Geometry: final body of the model. Coordinates: model frame, mm. A direction names the side the tool comes from. Round coordinates to 2 decimals unless told otherwise and drop trailing zeros. Loops run counter-clockwise (first coordinate to the right, second up) from the corner with the lowest first, then second, coordinate; pieces in that order, holes last. Notation, with made-up numbers: (41, 74) - (99, 74) arc R7 cw to (99, 82) - close; hole circle Ø8 at (-33.75, 52.25). An arc over 180 degrees is marked (long way). Return JSON: item names as keys, results as strings. Group by question number.
1. First-contact query: pin 1 Ø3.5 at (x, y) = (-2, 2.5) entering from -Z; pin 2 Ø0.5 at (y, z) = (6.5, -0.5) entering from -X. Flat tips, straight axial feed; report the tip coordinate or a pass-through.
2. Section B-B on x = -15. Return loops of the section in (y, z).
3. Set-up query: faces 1 (the face through (14.325, -1.312, 0.592)), 2 (the face through (0, 0, 0)), 3 (the face through (0, 0, 1.2)). Return all of +Z, -Z, +X, -X, +Y, -Y with unobstructed straight access to the full face (end or side cutting, diameter ignored); none if empty.
4. Draft query along X for faces 4 (the face through (-3, 5.817, 1)), 5 (the face through (-17.398, 5.697, 0.592)), 6 (the face through (-1, 6.717, 1)). Return one class per face: +X half, -X half, draft (parallel to the pull), parting line (faces both ways), or undercut.
5. Section A-A on x = 5. Return loops of the section in (y, z).
6. Section C-C on z = -1. Return loops of the section in (x, y), and give its area (3 significant figures).
7. Section D-D on y = -1.25. Return loops of the section in (x, z).
8. Material intervals for probe 1 along Y at (x, z) = (-9, 0.25); probe 2 along Y at (x, z) = (2, 2.5); probe 3 along Z at (x, y) = (9.5, -4.5), sorted ascending.
from build123d import *

# Parameters (mm, degrees)
EXTRUDE_1_DEPTH     = 1.2
CUT_EXTRUDE_START   = -1.2
CUT_EXTRUDE_1_DEPTH = 1.2
SKETCH_4_R          = 0.3
EXTRUDE_2_DEPTH     = 0.3
SKETCH_5_W          = 35.331764914
SKETCH_5_H          = 6.20328697
EXTRUDE_3_DEPTH     = 0.6


# Read off the part's stored shape, not the designer's step: Вырез-Вытянуть-Тонкостенный1
with BuildPart() as part:
    # Эскиз2 → Бобышка-Вытянуть1 (new body)
    with BuildSketch(Plane.XY):
        with BuildLine():
            Line((-18.718376773, 5.964639596), (-19.098029559, 5.834924894))
            Line((-19.098029559, 5.834924894), (-13.908113328, -6.217213911))
            Line((-13.908113328, -6.217213911), (10.163695982, -6.217213911))
            Line((10.163695982, -6.217213911), (19.098029559, 3.075246962))
            Line((19.098029559, 3.075246962), (18.818052215, 3.361181271))
            add(Edge.make_bspline(
                [(18.818052215, 3.361181271), (18.196335672, 3.797817809), (16.975433986, 4.6552669), (14.927683514, 5.553251977), (12.774537573, 6.124349252), (11.289757629, 6.1860932), (10.541386196, 6.217213911)],
                knots=[0, 0, 0, 0, 0.255164744, 0.501082157, 0.74853118, 1, 1, 1, 1], degree=3))
            Line((10.541386196, 6.217213911), (-16.231491208, 6.217213911))
            Line((-16.231491208, 6.217213911), (-18.718376773, 5.964639596))
        make_face()
    extrude(amount=EXTRUDE_1_DEPTH)

    # Вырез-Вытянуть-Тонкостенный1 outline → Вырез-Вытянуть-Тонкостенный1 (cut)
    with BuildSketch(Plane.XY.offset(1.2).offset(CUT_EXTRUDE_START)):
        with BuildLine():
            Line((19.098029559, 3.075246962), (18.818052215, 3.361181271))
            add(Edge.make_bspline(
                [(18.818052215, 3.361181271), (18.196335672, 3.797817809), (16.975433986, 4.6552669), (14.927683514, 5.553251977), (12.774537573, 6.124349252), (11.289757629, 6.1860932), (10.541386196, 6.217213911)],
                knots=[0, 0, 0, 0, 0.255164744, 0.501082157, 0.74853118, 1, 1, 1, 1], degree=3))
            Line((10.541386196, 6.217213911), (-16.231491208, 6.217213911))
            Line((-16.231491208, 6.217213911), (-18.718376773, 5.964639596))
            Line((-18.718376773, 5.964639596), (-19.098029559, 5.834924894))
            Line((-19.098029559, 5.834924894), (-13.908113328, -6.217213911))
            Line((-13.908113328, -6.217213911), (10.163695982, -6.217213911))
            Line((10.163695982, -6.217213911), (19.098029559, 3.075246962))
        make_face()
        with BuildLine():
            add(Edge.make_bspline(
                [(18.537521774, 3.069405939), (17.947435083, 3.483762917), (17.356771233, 3.89722808), (16.097834512, 4.604238585), (15.441178256, 4.89047439), (14.096932161, 5.359287166), (13.40761017, 5.542927998), (11.977353684, 5.757866724), (11.254825306, 5.787199054), (10.533072773, 5.817213911)],
                knots=[0, 0, 0, 0, 0.25, 0.25, 0.5, 0.5, 0.75, 0.75, 1, 1, 1, 1], degree=3))
            Line((18.537521774, 3.069405939), (9.993388288, -5.817213911))
            Line((9.993388288, -5.817213911), (-13.644851339, -5.817213911))
            Line((-13.644851339, -5.817213911), (-18.552496655, 5.5794291))
            Line((-18.552496655, 5.5794291), (-16.21123082, 5.817213911))
            Line((-16.21123082, 5.817213911), (10.533072773, 5.817213911))
        make_face(mode=Mode.SUBTRACT)
    extrude(amount=CUT_EXTRUDE_1_DEPTH, mode=Mode.SUBTRACT)

    # Эскиз4 → Бобышка-Вытянуть2 (add)
    with BuildSketch(Plane(origin=(0, 5.817213911, 0), x_dir=(1, 0, 0), z_dir=(0, 1, 0))):
        with Locations(Location((-15.91123082, -0.6, 0), (0, 0, 180))):
            Circle(SKETCH_4_R)
        with Locations(Location((-7.21123082, -0.6, 0), (0, 0, 270))):
            Circle(SKETCH_4_R)
        with Locations(Location((1.48876918, -0.6, 0), (0, 0, 270))):
            Circle(SKETCH_4_R)
        with Locations(Location((10.18876918, -0.6, 0), (0, 0, 270))):
            Circle(SKETCH_4_R)
    extrude(amount=EXTRUDE_2_DEPTH)

    # Эскиз5 → Бобышка-Вытянуть3 (add)
    with BuildSketch(Plane(origin=(0, 6.117213911, 0), x_dir=(1, 0, 0), z_dir=(0, 1, 0))):
        with Locations((-0.636806408, -0.824756774)):
            Rectangle(SKETCH_5_W, SKETCH_5_H)
    extrude(amount=EXTRUDE_3_DEPTH)


solid = part.part
Taken from the geometry:
{
 "1": {"pin 1": "z = 0", "pin 2": "x = -18.3"},
 "2": {"outline": "(-2.67, 0) - (5.82, 0) - (5.82, 1.2) - (-2.67, 1.2) - close; (6.12, -2.28) - (6.72, -2.28) - (6.72, 3.93) - (6.12, 3.93) - close"},
 "3": {"face 1": "+Z, -Z, +X, -Y", "face 2": "-Z, +X, -X, -Y", "face 3": "+Z, +X, -X, -Y"},
 "4": {"face 4": "undercut", "face 5": "-X half", "face 6": "draft"},
 "5": {"outline": "(-5.82, 0) - (5.82, 0) - (5.82, 1.2) - (-5.82, 1.2) - close; (6.12, -2.28) - (6.72, -2.28) - (6.72, 3.93) - (6.12, 3.93) - close"},
 "6": {"outline": "(-18.3, 6.12) - (17.03, 6.12) - (17.03, 6.72) - (-18.3, 6.72) - close", "area": "21.2 mm2"},
 "7": {"outline": "(-15.61, 0) - (14.38, 0) - (14.38, 1.2) - (-15.61, 1.2) - close"},
 "8": {"probe 1": "-5.82 to 5.82, 6.12 to 6.72", "probe 2": "6.12 to 6.72", "probe 3": "0 to 1.2"}
}
